Geometry: final body of the model. Coordinates: model frame, mm. Face numbers are marked on the shaded views. A direction names the side the tool comes from. Give positions to 0.01 mm unless a question says otherwise; leave off trailing zeros. Loops run counter-clockwise (first coordinate to the right, second up) from the corner with the lowest first, then second, coordinate; pieces in that order, holes last. Notation, with made-up numbers: (36.25, 35) - (45.25, 35) arc R28 ccw to (45.25, 58) - close; hole circle Ø3 at (21, 27). An arc over 180 degrees is marked (long way). Answer in a Markdown table with one row per item.
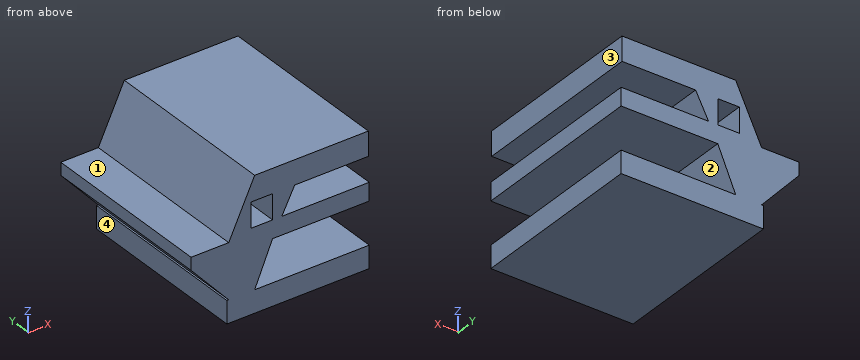
from build123d import *

# Parameters (mm, degrees)
F0_W     = 24.573456496
F0_H     = 8.1911524758
F0_W_2   = 74.8905315995
F0_H_2   = 14.6270543337
F0_W_3   = 48.7080998719
F0_H_3   = 11.7016462609
F1_DEPTH = 25.4
F2_DEPTH = 91.186


with BuildPart() as f1:
    # F0 (on Front) → F1 (new body)
    with BuildSketch(Plane.XZ):
        with Locations((-55.436545983, 4.0955762379)):
            Rectangle(F0_W, F0_H)
        Polygon((-26.1824317276, 43.8811704516), (-43.149817735, 8.1911524758), (-43.149817735, 0), (-67.723274231, 0), (-43.149817735, -27.4988673627), (-26.1824317276, -27.4988673627), (-14.4807854667, 0), (-28.5227615386, 0), (-28.5227615386, 11.7016462609), (-28.5227615386, 28.0839502811), (-14.4807854667, 28.0839502811), (-14.4807854667, 11.7016462609), (-12.1404575184, 11.7016462609), (-8.4471246955, 11.7016462609), (0, 28.0839502811), (48.1230206788, 28.0839502811), (48.1230206788, 43.8811704516), align=None)
        Polygon((-26.1824317276, -27.4988673627), (-43.149817735, -27.4988673627), (-44.3199835718, -27.4988673627), (-44.3199835718, -42.1259216964), (-26.1824317276, -42.1259216964), align=None)
        with Locations((11.2628340721, -34.8123945296)):
            Rectangle(F0_W_2, F0_H_2)
        Polygon((-28.5227615386, 0), (-14.4807854667, 0), (-12.1404575184, 4.5388182771), (-12.1404575184, 11.7016462609), (-14.4807854667, 11.7016462609), (-28.5227615386, 11.7016462609), align=None)
        Polygon((-12.1404575184, 4.5388182771), (-14.4807854667, 0), (-12.1404575184, 0), align=None)
        Polygon((-12.1404575184, 11.7016462609), (-12.1404575184, 4.5388182771), (-8.4471246955, 11.7016462609), align=None)
        Polygon((-8.4471246955, 11.7016462609), (-12.1404575184, 4.5388182771), (-12.1404575184, 0), (0, 0), (0, 11.7016462609), align=None)
        with Locations((24.3540499359, 5.8508231305)):
            Rectangle(F0_W_3, F0_H_3)
    extrude(amount=F1_DEPTH)

    # F2 (add): a face of the model
    f2_faces = [f1.faces().sort_by_distance(p)[0] for p in [
        (-55.436545983, -25.4, 6.7436206186),
    ]]
    extrude(f2_faces, amount=F2_DEPTH)


solid = f1.part
Q1. Cut plane A-A (y = -80.5). Output: boundary loops of the cut face in (x, z).
Check values:
| item | result |
|---|---|
| outline | (-67.72, 0) - (-43.15, -27.5) - (-44.32, -27.5) - (-44.32, -42.13) - (48.71, -42.13) - (48.71, -27.5) - (-26.18, -27.5) - (-14.48, 0) - (48.71, 0) - (48.71, 11.7) - (-8.45, 11.7) - (0, 28.08) - (48.12, 28.08) - (48.12, 43.88) - (-26.18, 43.88) - (-43.15, 8.19) - (-67.72, 8.19) - close; hole (-28.52, 11.7) - (-14.48, 11.7) - (-14.48, 28.08) - (-28.52, 28.08) - close |
Q2. Reachability of the marked faces 1, 2, 3 and 4 from +Z, -Z, +X, -X, +Y, -Y: full face, straight path, thin tool, end or side. Return the list, or none.
Check values:
| item | result |
|---|---|
| face 1 | +Z, -X, +Y, -Y |
| face 2 | +X, +Y, -Y |
| face 3 | +Z, +X, +Y, -Y |
| face 4 | -Z, -X, +Y, -Y |
Q3. Cut plane D-D (x = -20). Output: boundary loops of the cut face in (y, z).
Check values:
| item | result |
|---|---|
| outline | (-116.59, -42.13) - (0, -42.13) - (0, -27.5) - (-116.59, -27.5) - close; (-116.59, -12.97) - (0, -12.97) - (0, 11.7) - (-116.59, 11.7) - close; (-116.59, 28.08) - (0, 28.08) - (0, 43.88) - (-116.59, 43.88) - close |
Q4. Material intervals for line 1 along Z through (x, y) = (42.5, -64.5); line 2 along Z through (x, y) = (-2, -66); line 3 along X through (y, z) = (-91, 24), sorted ascending.
Check values:
| item | result |
|---|---|
| line 1 | -42.13 to -27.5, 0 to 11.7, 28.08 to 43.88 |
| line 2 | -42.13 to -27.5, 0 to 11.7, 24.21 to 43.88 |
| line 3 | -35.63 to -28.52, -14.48 to -2.11 |
Q5. First-contact query: pin 1 (4 mm diameter, centred on x = -34.5, z = -6, fed in from +Y); pin 2 (1 mm diameter, centred on y = -33, z = -26, fed in from -X); pin 3 (8 mm diameter, centred on y = -68.5, z = -9, fed in from +X); pin 4 (1 mm diameter, centred on y = -26.5, z = 30, fed in from -X). Flat tips, straight axial feed; report the tip coordinate or a pass-through.
Check values:
| item | result |
|---|---|
| pin 1 | y = 0 |
| pin 2 | x = -44.94 |
| pin 3 | x = -16.61 |
| pin 4 | x = -33.02 |
Q6. Cut plane C-C (z = 21). Output: boundary loops of the cut face in (x, y).
Check values:
| item | result |
|---|---|
| outline | (-37.06, -116.59) - (-28.52, -116.59) - (-28.52, 0) - (-37.06, 0) - close; (-14.48, -116.59) - (-3.65, -116.59) - (-3.65, 0) - (-14.48, 0) - close |
Q7. Cut plane B-B (x = 32). Output: boundary loops of the cut face in (y, z), and give its area (3 significant figures).
Check values:
| item | result |
|---|---|
| outline | (-116.59, -42.13) - (0, -42.13) - (0, -27.5) - (-116.59, -27.5) - close; (-116.59, 0) - (0, 0) - (0, 11.7) - (-116.59, 11.7) - close; (-116.59, 28.08) - (0, 28.08) - (0, 43.88) - (-116.59, 43.88) - close |
| area | 4,910 mm² |
